Verification items for the finished model (mm, model axes). Coordinates: 2 decimals unless noted, no trailing zeros. Loops run counter-clockwise (first coordinate to the right, second up) from the corner with the lowest first, then second, coordinate; pieces in that order, holes last. Notation, with made-up numbers: (-6, 45.5) -> (34, 45.5) arc R16 ccw to (34, 66.5) -> close; hole circle Ø11 at (80.25, -19.75). An arc over 180 degrees is marked (long way). Answer as a JSON object with one key per item and string values. Group by question number.
Q1. Cross-section at B-B on y = -457. Record the boundary of the cut face in (x, z), and give its area (3 significant figures).
Q2. Gauge pin test, flat end, axial feed: pin 1 Ø10 at (x, y) = (0, -424.5) entering from +Z. Record the tip position at first contact, or that the pin passes through.
Q3. Scan lines: L1, parallel to Y at x = 0, z = 0.55; L2, parallel to X at y = -2466.95, z = 0.8; L3, parallel to X at y = -325.5, z = 6.5. Record each from-to range of solid material in increasing order.
Q4. Cross-section at A-A on z = 6.75. Record the boundary of the cut face in (x, y), and give its area (3 significant figures).
```python
from build123d import *

# Parameters (mm, degrees)
PAD_DEPTH    = 2500
SKETCH_R     = 8
SKETCH_R_2   = 3.05
POCKET_DEPTH = 2.5


with BuildPart() as part:
    # Sketch002 → Pad (new body)
    with BuildSketch(Plane.XZ):
        Polygon((-20.5, 0), (-20.5, 21), (-10.5, 21), (-10.5, 14), (-13, 14), (-13, 18.5), (-18, 18.5), (-18, 2.5), (18, 2.5), (18, 18.5), (13, 18.5), (13, 14), (10.5, 14), (10.5, 21), (20.5, 21), (20.5, 0), align=None)
    extrude(amount=PAD_DEPTH)

    # Sketch (on Face10 of Pad) → Pocket (cut)
    with BuildSketch(Plane(origin=(0, 0, 2.5), x_dir=(-1, 0, 0), z_dir=(0, 0, 1))):
        with Locations((0, 30)):
            Circle(SKETCH_R)
        with Locations((0, 2466.95)):
            Circle(SKETCH_R_2)
        with Locations((0, 2396.95)):
            Circle(SKETCH_R_2)
    extrude(amount=-POCKET_DEPTH, mode=Mode.SUBTRACT)


solid = part.part
```
Computed values:
{
 "1": {"outline": "(-20.5, 0) -> (20.5, 0) -> (20.5, 21) -> (10.5, 21) -> (10.5, 14) -> (13, 14) -> (13, 18.5) -> (18, 18.5) -> (18, 2.5) -> (-18, 2.5) -> (-18, 18.5) -> (-13, 18.5) -> (-13, 14) -> (-10.5, 14) -> (-10.5, 21) -> (-20.5, 21) -> close", "area": "255 mm²"},
 "2": {"pin 1": "stops at z = 2.5"},
 "3": {"L1": "y = -2500 to -2470, -2463.9 to -2400, -2393.9 to -38, -22 to 0", "L2": "x = -20.5 to -3.05, 3.05 to 20.5", "L3": "x = -20.5 to -18, 18 to 20.5"},
 "4": {"outline": "(-20.5, -2500) -> (-18, -2500) -> (-18, 0) -> (-20.5, 0) -> close; (18, -2500) -> (20.5, -2500) -> (20.5, 0) -> (18, 0) -> close", "area": "12,500 mm²"}
}
